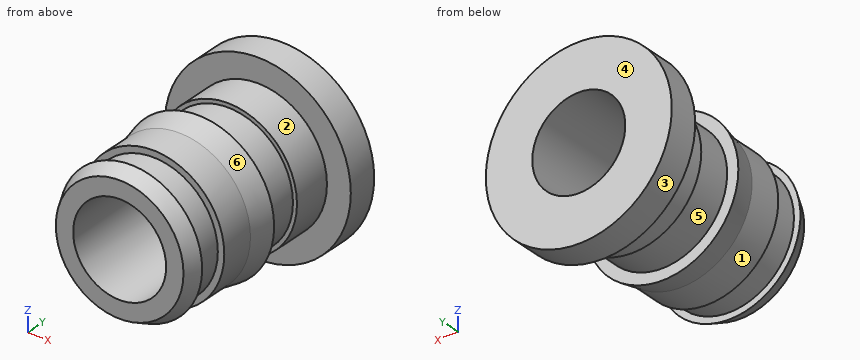
```python
from build123d import *

# Parameters (mm, degrees)
F0_R      = 9.525
F1_DEPTH  = 3.175
F2_R      = 7.08025
F3_DEPTH  = 4.064
F4_R      = 6.6675
F5_DEPTH  = 4.064
F6_R      = 7.8105
F7_DEPTH  = 2.54
F8_R      = 7.3025
F9_DEPTH  = 3.556
F10_R     = 6.6421
F11_DEPTH = 2.9972
F12_R     = 7.3025
F13_DEPTH = 1.524
F14_SIZE2 = 2.53999
F14_SIZE  = 0.50799
F15_SIZE2 = 1.52399
F15_SIZE  = 0.76199
F16_R     = 4.7625
F17_DEPTH = 21.9212


# Not quite as in the source:
# - a fillet or chamfer is up to 0.001 mm smaller than in the source, because OpenCascade refuses the exact size


with BuildPart() as f1:
    # F0 (on Front) → F1 (new body)
    with BuildSketch(Plane.XZ):
        Circle(F0_R)
    extrude(amount=F1_DEPTH)

    # F2 (on face) → F3 (join)
    with BuildSketch(Plane.XZ.offset(3.175)):
        Circle(F2_R)
    extrude(amount=F3_DEPTH)

    # F4 (on face) → F5 (join)
    with BuildSketch(Plane.XZ.offset(7.239)):
        Circle(F4_R)
    extrude(amount=F5_DEPTH)

    # F6 (on face) → F7 (join)
    with BuildSketch(Plane.XZ.offset(11.303)):
        Circle(F6_R)
    extrude(amount=F7_DEPTH)

    # F8 (on face) → F9 (join)
    with BuildSketch(Plane.XZ.offset(13.843)):
        Circle(F8_R)
    extrude(amount=F9_DEPTH)

    # F10 (on face) → F11 (join)
    with BuildSketch(Plane.XZ.offset(17.399)):
        Circle(F10_R)
    extrude(amount=F11_DEPTH)

    # F12 (on face) → F13 (join)
    with BuildSketch(Plane.XZ.offset(20.3962)):
        Circle(F12_R)
    extrude(amount=F13_DEPTH)

    # F14 (size 0.508 and 2.54 in the source; OpenCascade refuses exactly that, so slightly less here)
    f14_edges = [f1.edges().sort_by_distance(p)[0] for p in [
        (-7.8105, -13.843, 0),
    ]]
    f14_side = f1.faces().sort_by_distance((-7.589586, -13.843, 0))[0]
    chamfer(f14_edges, length=F14_SIZE, length2=F14_SIZE2, reference=f14_side)

    # F15 (size 0.762 and 1.524 in the source; OpenCascade refuses exactly that, so slightly less here)
    f15_edges = [f1.edges().sort_by_distance(p)[0] for p in [
        (-7.3025, -21.9202, 0),
    ]]
    f15_side = f1.faces().sort_by_distance((0, -21.9202, 0))[0]
    chamfer(f15_edges, length=F15_SIZE, length2=F15_SIZE2, reference=f15_side)

    # F16 (on face) → F17 (cut, through all)
    with BuildSketch(Plane.XZ.offset(21.9202)):
        Circle(F16_R)
    extrude(amount=-F17_DEPTH, mode=Mode.SUBTRACT)


solid = f1.part
```
Geometry check sheet. Reference: the model listing, model coordinates, mm. Face numbers are marked on the shaded views. A direction names the side the tool comes from. Give positions to 0.01 mm unless a question says otherwise; leave off trailing zeros. Order: outer loops, then holes, each group sorted by start corner. A loop starts at its lowest first (then second) coordinate and runs counter-clockwise, first axis right, second up. Notation, with made-up numbers: (52, 8.25) - (94, 8.25) arc R21 ccw to (94, 37.25) - close; hole circle Ø3 at (69, 80). An arc over 180 degrees is marked (long way). Answer in a Markdown table with one row per item. Add a question column.
Q1. Mould release check, pull along Y, two halves, no side actions. Record for the marked faces 4, 5 and 6: pulls with the +Y half, pulls with the -Y half, needs draft (parallel to the pull), parting line crosses it, or undercut.
Q2. Cross-section at B-B, the plane y = -19.25. Enter the section's corners in (x, z) (1 decimal).
Q3. Gauge pin test, flat ends, axial feed: pin 1 (3 mm diameter, centred on y = -7.5, z = -4, fed in from +X); pin 2 (10 mm diameter, centred on x = 4.5, y = -9.5, fed in from -Z); pin 3 (6 mm diameter, centred on x = 7, y = -3.5, fed in from -Z); pin 4 (11 mm diameter, centred on x = 0, z = 0, fed in from -Y). Record the tip position at first contact, or that the pin passes through.
Q4. Material ranges on probe 1 along Z at (x, y) = (0, -14.5); probe 2 along Z at (x, y) = (0, -6.75); probe 3 along Y at (x, z) = (-5.75, 7.25) (3 decimals), recorded low to high. Write a range as from..to.
Q5. Cross-section at A-A, the plane y = -15.5. Enter the section's corners in (x, z) (1 decimal), then the cut area to 3 significant figures.
Q6. Tool access check on the marked faces 1, 2 and 3. Record the directions out of +Z, -Z, +X, -X, +Y, -Y that give a thin tool (end or side, any length) a straight path to the whole face; none if there is none.
Check values:
| question | item | result |
|---|---|---|
| 1 | face 4 | pulls with the +Y half |
| 1 | face 5 | undercut |
| 1 | face 6 | pulls with the -Y half |
| 2 | outline | circle Ø13.3 at (0, 0); hole circle Ø9.5 at (0, 0) |
| 3 | pin 1 | stops at x = 6.62 |
| 3 | pin 2 | stops at z = -7.81 |
| 3 | pin 3 | stops at z = -8.64 |
| 3 | pin 4 | stops at y = -21.92 |
| 4 | probe 1 | z = -7.3..-4.76, 4.76..7.3 |
| 4 | probe 2 | z = -7.08..-4.76, 4.76..7.08 |
| 4 | probe 3 | y = -3.175..0 |
| 5 | outline | circle Ø14.6 at (0, 0); hole circle Ø9.5 at (0, 0) |
| 5 | area | 96.3 mm^2 |
| 6 | face 1 | -Y |
| 6 | face 2 | none |
| 6 | face 3 | +Y, -Y |
